```python
from build123d import *

# Parameters (mm, degrees)
F0_W      = 50.8
F0_H      = 50.8
F1_DEPTH  = 25.4
F1_FACE_W = 50.8
F1_FACE_H = 50.8
F3_T      = -2.54
F5_D      = 6.35


# Not quite as in the source:
# - a shell that OpenCascade refuses in one call is made with other operations: the cavity is built on its own and cut out


with BuildPart() as f1:
    # F0 (on Front) → F1 (new body, symmetric)
    with BuildSketch(Plane.XZ):
        Rectangle(F0_W, F0_H)
    extrude(amount=F1_DEPTH, both=True)

    # F1_face (on face) → F2 (revolve)
    with BuildSketch(Plane.XZ.offset(25.4)):
        Rectangle(F1_FACE_W, F1_FACE_H)
    revolve(axis=Axis((-25.4, -25.4, 0), (0, 0, 1)))

    # F3: a shell. OpenCascade refuses it in one call, so the cavity is built on its own and cut out:
    # the body offset inwards by the wall thickness, plus a prism from it out through each open face.
    f3_core = offset(f1.part, amount=F3_T, mode=Mode.PRIVATE)
    f3_exits = [f3_core.faces().sort_by_distance(p)[0] for p in [
        (22.86, -1.27, 0),
    ]]
    add(f3_core, mode=Mode.SUBTRACT)
    extrude(f3_exits, amount=-F3_T, mode=Mode.SUBTRACT)

    # F5 (through all)
    with Locations(Plane(origin=(0, 25.4, 0), x_dir=(-1, 0, 0), z_dir=(0, 1, 0))):
        with Locations((0, 12.914407067), (0, -15.8760398626)):
            Hole(F5_D / 2)


solid = f1.part
```
Geometry check sheet. Reference: the model listing, model coordinates, mm. A direction names the side the tool comes from. Round coordinates to 2 decimals unless told otherwise and drop trailing zeros. Loops run counter-clockwise (first coordinate to the right, second up) from the corner with the lowest first, then second, coordinate; pieces in that order, holes last. Notation, with made-up numbers: (74, -30.5) - (81, -30.5) arc R21 cw to (81, -23.5) - close; hole circle Ø4 at (-3.75, -23.5). An arc over 180 degrees is marked (long way). Use a Markdown table: item, result.
Q1. Go/stop test with flat-tipped pins: P1, Ø7.5, axis at x = 0, z = 12.91, coming from the +Y side; P2, Ø4, axis at x = -23.5, z = -2.5, coming from the -Y side; P3, Ø10, axis at x = 0, z = -15.88, coming from the -Y side; P4, Ø13.5, axis at x = 8, z = -1.5, coming from the -Y side. Record where each tip stops, or that it passes through.
Solutions:
| item | result |
|---|---|
| P1 | stops at y = 25.4 |
| P2 | stops at y = -76.2 |
| P3 | stops at y = -71.92 |
| P4 | stops at y = -68.65 |
Q2. Cross-section at B-B on z = -3. Record the cut outline in (x, y), plus the area to 3 significant figures.
Solutions:
| item | result |
|---|---|
| outline | (-25.4, 22.86) - (25.4, 22.86) - (25.4, 25.4) - (-25.4, 25.4) arc R50.8 ccw (long way) to (25.4, -25.4) - (22.86, -25.4) arc R48.26 cw (long way) to start |
| area | 722 mm2 |
Q3. Cross-section at A-A on x = 0. Record the cut outline in (y, z).
Solutions:
| item | result |
|---|---|
| outline | (-69.39, -25.4) - (25.4, -25.4) - (25.4, -19.05) - (22.86, -19.05) - (22.86, -22.86) - (-66.43, -22.86) - (-66.43, -19.05) - (-69.39, -19.05) - close; (-69.39, -12.7) - (-66.43, -12.7) - (-66.43, 9.74) - (-69.39, 9.74) - close; (-69.39, 16.09) - (-66.43, 16.09) - (-66.43, 22.86) - (22.86, 22.86) - (22.86, 16.09) - (25.4, 16.09) - (25.4, 25.4) - (-69.39, 25.4) - close; (22.86, -12.7) - (25.4, -12.7) - (25.4, 9.74) - (22.86, 9.74) - close |
Q4. Cross-section at C-C on x = -52.5. Record the cut outline in (y, z).
Solutions:
| item | result |
|---|---|
| outline | (-68.37, -25.4) - (17.57, -25.4) - (17.57, 25.4) - (-68.37, 25.4) - close; hole (-65.33, -22.86) - (14.53, -22.86) - (14.53, 22.86) - (-65.33, 22.86) - close |
Q5. Access from +Z, -Z, +X, -X, +Y, -Y to the whole of each face (thin tool, end or side, straight path). Record for faces 4 (the flat face through (24, -25.4, 0)), 5 (the cylindrical face through (-60.632, -58.381, 0.32)), 6 (the cylindrical face through (-0.413, 24.112, -12.728)).
Solutions:
| item | result |
|---|---|
| face 4 | +X |
| face 5 | none |
| face 6 | +Y, -Y |
Q6. Material ranges on line 1 (Z direction, x = 0, y = -67); line 2 (Z direction, x = 0, y = -66); line 3 (Y direction, x = -27, z = 15.5), recorded low to high.
Solutions:
| item | result |
|---|---|
| line 1 | z = -25.4 to -19.05, -12.7 to 9.74, 16.09 to 25.4 |
| line 2 | z = -25.4 to -22.86, 22.86 to 25.4 |
| line 3 | y = -76.17 to -73.63, 22.83 to 25.37 |
Q7. Draft check along Z on faces 1 (the flat face through (25.4, 24, 0)), 2 (the flat face through (-25, -25, 25.4)), 3 (the cylindrical face through (1.71, -67.75, 15.59)). Enter one of: released by +Z, released by -Z, zero draft, split by the parting line, or undercut.
Solutions:
| item | result |
|---|---|
| face 1 | zero draft |
| face 2 | released by +Z |
| face 3 | undercut |
Q8. Cross-section at D-D on y = -33. Record the cut outline in (x, z), plus the area to 3 significant figures.
Solutions:
| item | result |
|---|---|
| outline | (-75.63, -25.4) - (24.83, -25.4) - (24.83, 25.4) - (-75.63, 25.4) - close; hole (-73.06, -22.86) - (22.26, -22.86) - (22.26, 22.86) - (-73.06, 22.86) - close |
| area | 745 mm2 |
